Input: part model. Units: mm. Frame: model coordinates. A direction names the side the tool comes from. Coordinates: 2 decimals unless noted, no trailing zeros. Write each loop counter-clockwise with the first axis right and the second up, starting at its lowest first coordinate (ties: lowest second). Pieces come first, ordered by that corner, then holes. Notation, with made-up numbers: (50.5, -30) - (67.5, -30) arc R20 ccw to (67.5, -20) - close; hole circle Ø5 at (15.5, 63). An arc over 180 degrees is marked (long way). One line per question, with ' | ' between items. Start each with the question number.
1) First-contact query: P1, Ø1.5, axis at y = -10.5, z = -0.5, coming from the +X side; P2, Ø3, axis at x = 0, z = 0, coming from the -Y side; P3, Ø10, axis at y = -13, z = -12.5, coming from the +X side; P4, Ø6, axis at x = -15.11, z = 8.72, coming from the +Y side. Flat tips, straight axial feed; report the tip coordinate or a pass-through.
2) Draft query along Z for faces 1 (the flat face through (0, 0, -3)), 2 (the cylindrical face through (-10.74, -2.46, -2.38)), 3 (the cylindrical face through (0.114, -6.134, -20.047)). Return one class per face: released by +Z, released by -Z, zero draft, split by the parting line, or undercut.
3) Section query C-C on x = 17. Return loops of the section in (y, z).
4) Reachability of faces 4 (the flat face through (-5, -7.3, -10)), 5 (the cylindrical face through (15.038, -6.134, -16.399)), 6 (the flat face through (-5, -5, -10)) from +Z, -Z, +X, -X, +Y, -Y: full face, straight path, thin tool, end or side. Return the list, or none.
5) Section query D-D on y = -16. Return loops of the section in (x, z).
6) Section query B-B on x = 0. Return loops of the section in (y, z).
7) Section query A-A on z = 0. Return loops of the section in (x, y), and give its area (3 significant figures).
8) Line query: line 1 (X direction, y = -12.5, z = 0); line 2 (X direction, y = -5.5, z = 9); line 3 (Y direction, x = 10, z = -17.5). Output: solid intervals per line, ascending.
```python
from build123d import *

# Parameters (mm, degrees)
SKETCH_1_R          = 11
EXTRUDE_1_DEPTH     = 19
SKETCH_2_R          = 22.25
EXTRUDE_2_DEPTH     = 2.3
SKETCH_3_R          = 2.6
CUT_EXTRUDE_1_DEPTH = 35.440165505
SKETCH_4_R          = 2.5
CUT_EXTRUDE_2_DEPTH = 37.757652265


with BuildPart() as part:
    # 草图1 → 凸台-拉伸1 (new body)
    with BuildSketch(Plane(origin=(0, 0, 0), x_dir=(1, 0, 0), z_dir=(0, 1, 0))):
        with Locations(Location((0, 0, 0), (0, 0, 270))):
            Circle(SKETCH_1_R)
    extrude(amount=-EXTRUDE_1_DEPTH)

    # 草图2 → 凸台-拉伸2 (add)
    with BuildSketch(Plane(origin=(0, -5, 0), x_dir=(1, 0, 0), z_dir=(0, 1, 0))):
        with Locations(Location((0, 0, 0), (0, 0, 270))):
            Circle(SKETCH_2_R)
    extrude(amount=-EXTRUDE_2_DEPTH)

    # 草图3 → 切除-拉伸1 (cut, through all)
    with BuildSketch(Plane(origin=(0, -5, 0), x_dir=(1, 0, 0), z_dir=(0, 1, 0))):
        with Locations(Location((0, 17.45, 0), (0, 0, 270))):
            Circle(SKETCH_3_R)
        with Locations(Location((15.112143296, -8.725, 0), (0, 0, 270))):
            Circle(SKETCH_3_R)
        with Locations(Location((-15.112143296, -8.725, 0), (0, 0, 270))):
            Circle(SKETCH_3_R)
    extrude(amount=-CUT_EXTRUDE_1_DEPTH, mode=Mode.SUBTRACT)

    # 草图4 → 切除-拉伸2 (cut, through all)
    with BuildSketch(Plane(origin=(0, 0, 0), x_dir=(1, 0, 0), z_dir=(0, 1, 0))):
        with Locations(Location((0, 0, 0), (0, 0, 270))):
            Circle(SKETCH_4_R)
    extrude(amount=-CUT_EXTRUDE_2_DEPTH, mode=Mode.SUBTRACT)


solid = part.part
```
Answer key:
1) P1: x = 11 | P2: through | P3: x = 8.05 | P4: y = -5
2) face 1: zero draft | face 2: split by the parting line | face 3: undercut
3) outline: (-7.3, -14.35) - (-5, -14.35) - (-5, 6.94) - (-7.3, 6.94) - close; (-7.3, 10.51) - (-5, 10.51) - (-5, 14.35) - (-7.3, 14.35) - close
4) face 4: -Y | face 5: +Y, -Y | face 6: +Y
5) outline: circle Ø22 at (0, 0); hole circle Ø5 at (0, 0)
6) outline: (-19, -11) - (-7.3, -11) - (-7.3, -14.85) - (-5, -14.85) - (-5, -11) - (0, -11) - (0, -2.5) - (-19, -2.5) - close; (-19, 2.5) - (0, 2.5) - (0, 11) - (-5, 11) - (-5, 22.25) - (-7.3, 22.25) - (-7.3, 11) - (-19, 11) - close; (-7.3, -22.25) - (-5, -22.25) - (-5, -20.05) - (-7.3, -20.05) - close
7) outline: (-22.25, -7.3) - (-11, -7.3) - (-11, -19) - (-2.5, -19) - (-2.5, 0) - (-11, 0) - (-11, -5) - (-22.25, -5) - close; (2.5, -19) - (11, -19) - (11, -7.3) - (22.25, -7.3) - (22.25, -5) - (11, -5) - (11, 0) - (2.5, 0) - close | area: 375 mm²
8) line 1: -11 to -2.5, 2.5 to 11 | line 2: -20.35 to -17.7, -12.53 to 12.53, 17.7 to 20.35 | line 3: -7.3 to -5
